Study the drawing (mm; zero at the part's minimum x, y, z) and answer. A direction names the side the tool comes from. Round coordinates to 2 decimals unless told otherwise and drop trailing zeros. Write each loop counter-clockwise with the first axis right and the second up, starting at its lowest first coordinate (ties: lowest second). Pieces come first, ordered by that corner, then holes.
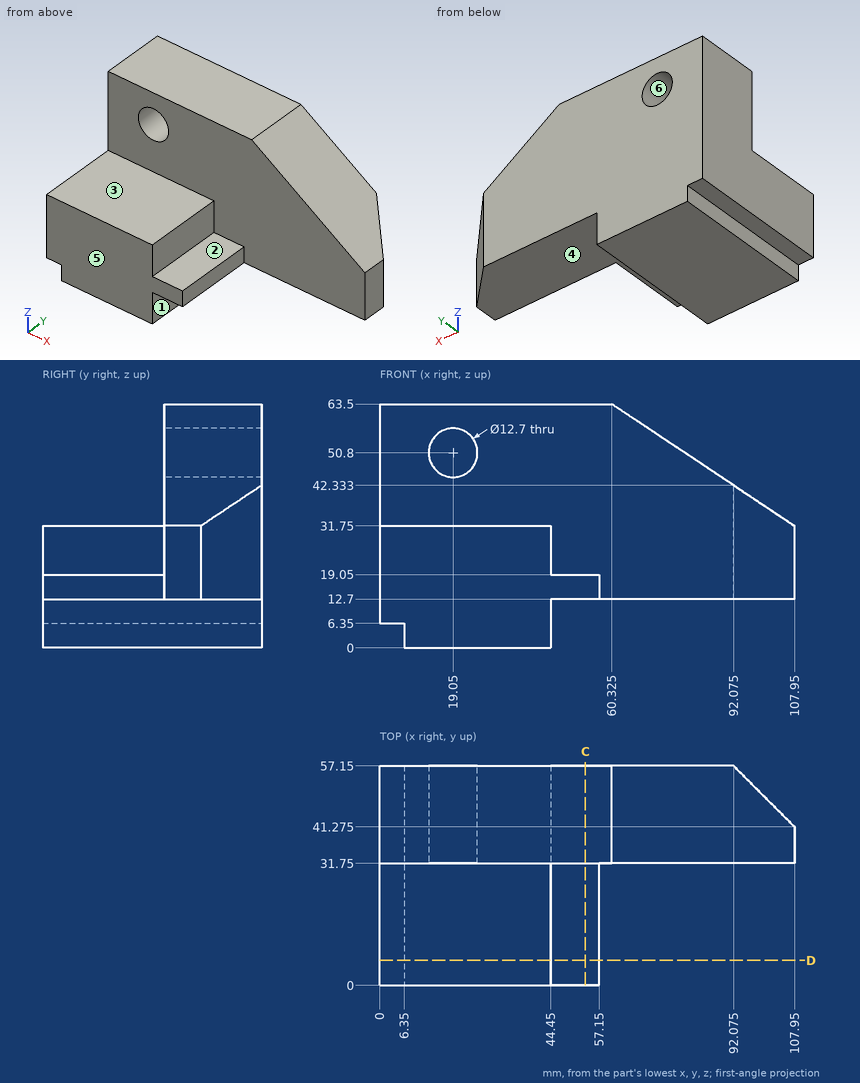
Q1. Given pin 1 (16.5 mm diameter, centred on x = 19.05, z = 50.8, fed in from -Y); pin 2 (2 mm diameter, centred on x = 85, y = 50.5, fed in from +Z); pin 3 (6.5 mm diameter, centred on y = 19, z = 8, fed in from +X), each flat-ended and moving along its own axis, determine where each tip first touches the part or whether it passes through.
Q2. A tool of negligible diameter and unlimited length cuts with its end or side. For the marked faces 1, 2 and 3, from which of +Z, -Z, +X, -X, +Y, -Y can it reach the whole face along a straight path? Write none if from no direction.
Q3. Find the intervals of material crossed by L1, parallel to Z at x = 17.5, y = 28.5; L2, parallel to Y at x = 47.5, z = 32; L3, parallel to Z at x = 47, y = 41, in increasing order.
Q4. The mould has two halves that part along Z. Classify the marked faces 4, 5 and 6: +Z half, -Z half, draft (parallel to the pull), parting line (faces both ways), or undercut.
Q5. Find section D-D (y = 6.5). Determine the outline of the cut face in (x, z).
Q6. Find section C-C (x = 53.5). Determine the outline of the cut face in (y, z), plus the area to 3 significant figures.
Report:
1. pin 1: stops at y = 31.75
1. pin 2: stops at z = 47.72
1. pin 3: stops at x = 44.45
2. face 1: -Z, +X, +Y, -Y
2. face 2: +Z, +X, -Y
2. face 3: +Z, +X, -X, -Y
3. L1: z = 0 to 31.75
3. L2: y = 31.75 to 57.15
3. L3: z = 12.7 to 63.5
4. face 4: -Z half
4. face 5: draft
4. face 6: undercut
5. outline: (0, 6.35) - (6.35, 6.35) - (6.35, 0) - (44.45, 0) - (44.45, 12.7) - (57.15, 12.7) - (57.15, 19.05) - (44.45, 19.05) - (44.45, 31.75) - (0, 31.75) - close
6. outline: (0, 12.7) - (57.15, 12.7) - (57.15, 63.5) - (31.75, 63.5) - (31.75, 19.05) - (0, 19.05) - close
6. area: 1,490 mm2
